from build123d import *

# Parameters (mm, degrees)
F2_R     = 14.024247
F0_DEPTH = 76.2
F1_T     = -2.54
F3_SIZE  = 2.032


with BuildPart() as f0:
    # F2 (on Front) → F0 (new body)
    with BuildSketch(Plane.XZ):
        Circle(F2_R)
    extrude(amount=F0_DEPTH)

    # F1
    f1_openings = [f0.faces().sort_by_distance(p)[0] for p in [
        (0, -76.2, 0),
    ]]
    offset(amount=F1_T, openings=f1_openings)

    # F3
    f3_edges = [f0.edges().sort_by_distance(p)[0] for p in [
        (-14.024247, 0, 0),
    ]]
    chamfer(f3_edges, length=F3_SIZE)


solid = f0.part
Geometry check sheet. Reference: the model listing, model coordinates, mm. A direction names the side the tool comes from. Give positions to 0.01 mm unless a question says otherwise; leave off trailing zeros. Loops run counter-clockwise (first coordinate to the right, second up) from the corner with the lowest first, then second, coordinate; pieces in that order, holes last.
(1) Depth check by flat-ended pin: pin 1 Ø1 at (x, z) = (-4.5, 11) entering from +Y; pin 2 Ø1.5 at (y, z) = (-22, 9) entering from -X; pin 3 Ø3 at (x, y) = (3, -52.5) entering from +Z; pin 4 Ø8 at (y, z) = (-9, -4.5) entering from +X. Enter the tip coordinate at first touch or a pass-through.
From the geometry:
pin 1: stops at y = 0
pin 2: stops at x = -11.34
pin 3: stops at z = 13.94
pin 4: stops at x = 14.02
(2) Section check A-A on x = 0. Record the cut outline in (y, z), then the cut area to 3 significant figures.
From the geometry:
outline: (-76.2, -14.02) - (-2.03, -14.02) - (0, -11.99) - (0, 11.99) - (-2.03, 14.02) - (-76.2, 14.02) - (-76.2, 11.48) - (-2.54, 11.48) - (-2.54, -11.48) - (-76.2, -11.48) - close
area: 441 mm2
(3) Release check for a two-part mould opening along Z. For faces 1 (the cylindrical face through (-3, -38.6, -13.7)), 2 (the flat face through (-11.5, -76.2, 2.1)), 3 (the flat face through (0, -2.54, 0)) record: released by +Z, released by -Z, zero draft, split by the parting line, or undercut.
From the geometry:
face 1: split by the parting line
face 2: zero draft
face 3: undercut
(4) Thickness scan on L1, parallel to Z at x = 0, y = -37; L2, parallel to Y at x = 5, z = 6. Record the ranges inside material, lowest first.
From the geometry:
L1: z = -14.02 to -11.48, 11.48 to 14.02
L2: y = -2.54 to 0
(5) Section check C-C on y = -48.5. Record the cut outline in (x, z), then the cut area to 3 significant figures.
From the geometry:
outline: circle Ø28.05 at (0, 0); hole circle Ø22.97 at (0, 0)
area: 204 mm2
(6) Set-up check for faces 4 (the flat face through (0, 0, 0)), 5 (the cylindrical face through (6.174, -38.854, 9.684)): record each of +Z, -Z, +X, -X, +Y, -Y from which the full face is reachable in a straight line by a thin tool's end or side.
From the geometry:
face 4: +Z, -Z, +X, -X, +Y
face 5: -Y
(7) Section check B-B on z = 0. Record the cut outline in (x, y), then the cut area to 3 significant figures.
From the geometry:
outline: (-14.02, -76.2) - (-11.48, -76.2) - (-11.48, -2.54) - (11.48, -2.54) - (11.48, -76.2) - (14.02, -76.2) - (14.02, -2.03) - (11.99, 0) - (-11.99, 0) - (-14.02, -2.03) - close
area: 441 mm2
